Read the model definition and answer for the solid it produces. Units are mm, in the model's axes. Face numbers are marked on the shaded views. A direction names the side the tool comes from. Round coordinates to 2 decimals unless told otherwise and drop trailing zeros. Order: outer loops, then holes, each group sorted by start corner. A loop starts at its lowest first (then second) coordinate and runs counter-clockwise, first axis right, second up. Notation, with made-up numbers: (68, 75.5) - (85, 75.5) arc R12 ccw to (85, 85.5) - close; hole circle Ø5 at (29.5, 46). An arc over 180 degrees is marked (long way). Put each result on its own line as item: value. Start each with the question number.
Q1. Find the intervals of material crossed by line 1 along X through (y, z) = (-12, 0); line 2 along Z through (x, y) = (7.5, -1.25); line 3 along X through (y, z) = (-9.75, -2.75), in increasing order. Write a range as from..to.
Q2. Each of these flat-tipped pins is pushed along its axis until it touches: pin 1 Ø5 at (x, y) = (-5.5, -12) entering from -Z; pin 2 Ø2.5 at (x, y) = (-2.5, -4) entering from +Z; pin 3 Ø6.5 at (x, y) = (0, -8.2) entering from +Z. Where does it stop, or does it pass through?
Q3. Section D-D on x = 2.5 is taken. Give the vertices of the cut face in (y, z), then the cut area to 3 significant figures.
Q4. Section A-A on z = 0 is taken. Give the vertices of the cut face in (x, y), then the cut area to 3 significant figures.
Q5. Which of the six approach directions +Z, -Z, +X, -X, +Y, -Y give full straight-line access (tool end or side, diameter ignored) to the marked faces 4 and 5?
Q6. For a pull along X with two mould halves and no side action, classify the marked faces 1, 2 and 3 as pulls with the +X half, pulls with the -X half, needs draft (parallel to the pull), parting line crosses it, or undercut.
Q7. Section B-B on x = 5.75 is taken. Give the vertices of the cut face in (y, z).
Q8. Section C-C on x = 0 is taken. Give the vertices of the cut face in (y, z).
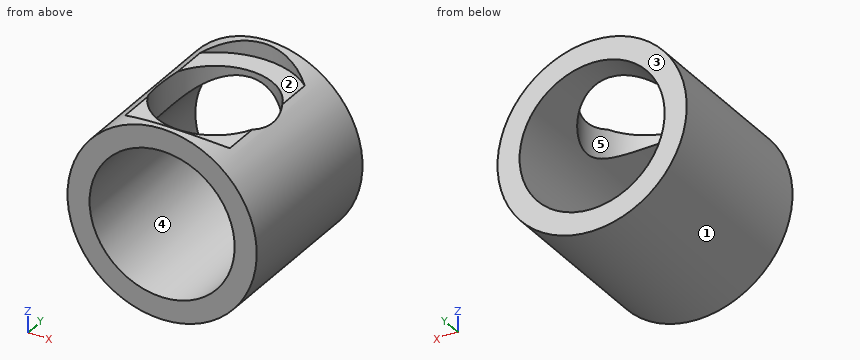
from build123d import *

# Parameters (mm, degrees)
SKETCH1_R               = 9
SKETCH1_R_2             = 6.9
BOSS_EXTRUDE1_DEPTH     = 16.4
CUT_EXTRUDE5_START      = 7.5
SKETCH3_R               = 7.65
CUT_EXTRUDE5_DEPTH      = 14.259576104
CUT_EXTRUDE6_DEPTH      = 25.944137756
CUT_EXTRUDE6_DEPTH_BACK = 7
SKETCH6_R               = 5.5


with BuildPart() as part:
    # Sketch1 → Boss-Extrude1 (new body)
    with BuildSketch(Plane(origin=(0, 0, 0), x_dir=(1, 0, 0), z_dir=(0, 1, 0))):
        with Locations(Location((0, 0, 0), (0, 0, 270))):
            Circle(SKETCH1_R)
        with Locations(Location((0, 0, 0), (0, 0, 270))):
            Circle(SKETCH1_R_2, mode=Mode.SUBTRACT)
    extrude(amount=-BOSS_EXTRUDE1_DEPTH)

    # Sketch3 → Cut-Extrude5 (cut, through all)
    with BuildSketch(Plane.XY.offset(CUT_EXTRUDE5_START)):
        with Locations((0, -8.2)):
            Circle(SKETCH3_R)
    extrude(amount=CUT_EXTRUDE5_DEPTH, mode=Mode.SUBTRACT)

    # Sketch6 → Cut-Extrude6 (cut, two sides: drawn at the far end of the back side and taken through both)
    with BuildSketch(Plane.XY.offset(7.5).offset(-CUT_EXTRUDE6_DEPTH_BACK)):
        with Locations(Location((0, -8.2, 0), (0, 0, 205.239401821))):
            Circle(SKETCH6_R)
    extrude(amount=CUT_EXTRUDE6_DEPTH + CUT_EXTRUDE6_DEPTH_BACK, mode=Mode.SUBTRACT)


solid = part.part
Findings:
1. line 1: -9..-6.9, 6.9..9
1. line 2: -4.97..4.97
1. line 3: -8.57..-6.33, 6.33..8.57
2. pin 1: z = -8.49
2. pin 2: z = 7.5
2. pin 3: z = -6.09
3. outline: (-16.4, -8.65) - (0, -8.65) - (0, -6.43) - (-16.4, -6.43) - close; (-16.4, 6.43) - (-13.1, 6.43) - (-13.1, 7.5) - (-15.43, 7.5) - (-15.43, 8.65) - (-16.4, 8.65) - close; (-3.3, 6.43) - (0, 6.43) - (0, 8.65) - (-0.97, 8.65) - (-0.97, 7.5) - (-3.3, 7.5) - close
3. area: 45.6 mm2
4. outline: (-9, -16.4) - (-6.9, -16.4) - (-6.9, 0) - (-9, 0) - close; (6.9, -16.4) - (9, -16.4) - (9, 0) - (6.9, 0) - close
4. area: 68.9 mm2
5. face 4: +Y, -Y
5. face 5: +Z
6. face 1: parting line crosses it
6. face 2: undercut
6. face 3: needs draft
7. outline: (-16.4, -6.92) - (0, -6.92) - (0, -3.81) - (-16.4, -3.81) - close; (-16.4, 3.81) - (0, 3.81) - (0, 6.92) - (-16.4, 6.92) - close
8. outline: (-16.4, -9) - (0, -9) - (0, -6.9) - (-16.4, -6.9) - close; (-16.4, 6.9) - (-13.7, 6.9) - (-13.7, 7.5) - (-15.85, 7.5) - (-15.85, 9) - (-16.4, 9) - close; (-2.7, 6.9) - (0, 6.9) - (0, 9) - (-0.55, 9) - (-0.55, 7.5) - (-2.7, 7.5) - close
